Design review of the part built by this model. Coordinates are the model's own, in mm. A direction names the side the tool comes from. Coordinates: 2 decimals unless noted, no trailing zeros. Loops run counter-clockwise (first coordinate to the right, second up) from the corner with the lowest first, then second, coordinate; pieces in that order, holes last. Notation, with made-up numbers: (64.25, -2) - (109.25, -2) arc R28 cw to (109.25, 31) - close; hole circle Ø3 at (81, 63.25). An arc over 180 degrees is marked (long way). Use one line per item in the form item = value. Start each with the question number.
(1) Clearance check with flat-ended pins moving along their axes: pin 1 Ø1.3 at (x, y) = (-11.93, 18.67) entering from -Z; pin 2 Ø0.6 at (x, z) = (4.5, 1) entering from -Y; pin 3 Ø2 at (x, y) = (7.5, -21) entering from -Z. State where each tip first meets the part, or that it passes through.
(2) Add section D-D (y = -56.75). State the section outline as (x, z) points.
(3) Add section B-B (z = 0.55). Count the separate pieces of the cut face and the enclosed holes in it, plus the area to 3 significant figures.
(4) Tool access review of faces 5 (the face through (8.1, -19.5, 1.5)), 6 (the face through (-8.41, -5.83, 1.01)), 7 (the face through (-15.75, -11, 1)): name each direction out of +Z, -Z, +X, -X, +Y, -Y from which nothing blocks a thin tool from reaching the whole face with its end or side.
(5) Add section A-A (y = 10.65). State the section outline as (x, z) points, plus the area to 3 significant figures.
(6) The part is to be moulded in two halves that separate along Y. For faces 1 (the face through (10.655, -49.735, 1.493)), 2 (the face through (15.75, -10, 1)), 3 (the face through (-7, 11.5, 1)), 4 (the face through (0.22, 19.25, 0.99)), say which applies: pulls with the +Y half, pulls with the -Y half, needs draft (parallel to the pull), parting line crosses it, or undercut.
(7) For L1, parallel to X at y = 10.5, z = 1.8; L2, parallel to X at y = -40.5, z = 0.5; L3, parallel to Y at x = -3.5, z = 1.3, list the stretches that pass through material, from the lowest coordinate up.
Autodesk Inventor part; units mm, degrees
ref_plane "YZ Plane" through (0, 0, 0) normal (1, 0, 0) x (0, 1, 0)
ref_plane "XZ Plane" through (0, 0, 0) normal (0, 1, 0) x (-1, 0, 0)
ref_plane "XY Plane" through (0, 0, 0) normal (0, 0, 1) x (1, 0, 0)
sketch "スケッチ1" plane through (0, 0, 0) normal (0, 0, 1) x (1, 0, 0)
  circle A0 centre (-10.8253, -50.5) radius 0.7835
  circle A1 centre (0, -56.75) radius 0.7835
  circle A2 centre (10.8253, -50.5) radius 0.7835
  circle A3 centre (11.9284, 18.6695) radius 0.7835
  circle A4 centre (0, 16.025) radius 0.7835
  circle A5 centre (-11.9284, 18.6695) radius 0.7835
  line L0 (-9.85, -18.05) -> (-9.85, -7.35)
  arc A6 (-6.8, 12.8) -> (-9.85, 9.75) centre (-6.8, 9.75) ccw
  line L1 (-6.8, 12.8) -> (6.8, 12.8)
  arc A7 (9.85, 9.75) -> (6.8, 12.8) centre (6.8, 9.75) ccw
  line L2 (9.85, 9.75) -> (9.85, 8.57)
  arc A8 (4.8, -23.1) -> (9.85, -18.05) centre (4.8, -18.05) ccw
  line L3 (4.8, -23.1) -> (-4.8, -23.1)
  arc A9 (-9.85, -18.05) -> (-4.8, -23.1) centre (-4.8, -18.05) ccw
  circle A10 centre (0, -44.25) radius 4
  arc A11 (-15.75, 24.8351) -> (15.75, 24.8351) centre (0, 44.25) ccw
  line L4 (-15.75, -44.25) -> (-15.75, 24.8351)
  arc A12 (-15.75, -44.25) -> (15.75, -44.25) centre (0, -44.25) ccw
  line L5 (15.75, 24.8351) -> (15.75, -44.25)
  line L6 (-9.85, 8.57) -> (9.85, 8.57)
  line L7 (9.85, 8.57) -> (9.85, -7.35)
  line L8 (9.85, -7.35) -> (-9.85, -7.35)
  line L9 (-9.85, -7.35) -> (-9.85, 8.57)
  line L10 (9.85, 8.57) -> (9.85, -7.35)
  line L11 (-9.85, 8.57) -> (-9.85, 9.75)
  line L12 (-9.85, -7.35) -> (-9.85, 8.57)
  line L13 (9.85, -7.35) -> (9.85, -18.05)
  point P0 (0, 0)
  point P1 (0, 0)
  dimension "d3" = 4.23
  dimension "d4" = 15.75
extrude "押し出し2" add sketch "スケッチ1" along normal blind 2 contours L0 L8 L13 A8 L3 A9 | L11 A6 L1 A7 L2 L6 | A11 L5 A12 L4
sketch "スケッチ2" plane through (0, 0, 2) normal (0, 0, 1) x (1, 0, 0)
  line L0 (9.85, -7.35) -> (-9.85, -7.35)
  line L1 (15.75, 24.8351) -> (15.75, -44.25)
  line L2 (-15.75, -44.25) -> (-15.75, 24.8351)
  line L3 (0, 18.6695) -> (0, -60)
  point P0 (0, 0)
  point P1 (0, 0)
  point P2 (-7.7, 10.65)
  point P3 (-7.2, -20.45)
  point P4 (7.2, -20.45)
  point P5 (7.7, 10.65)
  point P6 (0, -14.25)
  dimension "d10" = 31.1
  dimension "d11" = 31.1
  dimension "d12" = 15.4
  dimension "d13" = 14.4
  dimension "d14" = 15.4
  dimension "d15" = 31.5
  dimension "d16" = 14.4
  dimension "d26" = 6.9
  dimension "d27" = 6.2
  dimension "d28" = 6.2
hole "Hole2" at (7.7, 10.65, 2) at (7.2, -20.45, 2) at (-7.2, -20.45, 2) at (-7.7, 10.65, 2) at (0, -14.25, 2) direction (0, 0, -1) diameter 2.2 depth 8 tip angle 118
sketch "スケッチ4" plane through (0, 0, 2) normal (0, 0, 1) x (1, 0, 0)
  point P0 (0, 0)
  point P1 (0, -14.25)
hole "Hole3" at (0, -14.25, 2) direction (0, 0, -1) diameter 9 depth 8 tip angle 118
fillet "フィレット3" radius 1.05 2 edges at (-9.85, 8.57, 1) (9.85, 8.57, 1)
fillet "フィレット4" radius 5.05 2 edges at (-9.85, -7.35, 1) (9.85, -7.35, 1)
sketch "スケッチ6" plane through (0, 0, 0) normal (0, 0, -1) x (-1, 0, 0)
  circle A0 centre (-10.8253, -50.5) radius 0.7835
  circle A1 centre (0, -56.75) radius 0.7835
  circle A2 centre (10.8253, -50.5) radius 0.7835
  circle A3 centre (0, -44.25) radius 10.5
  circle A4 centre (0, -44.25) radius 14.5
  point P0 (0, 0)
  dimension "d50" = 21
  dimension "d51" = 29
extrude "押し出し4" cut sketch "スケッチ6" against normal blind 1
fillet "フィレット5" radius 0.5 2 edges at (-15.75, 24.8351, 1) (15.75, 24.8351, 1)
sketch "スケッチ8" plane through (0, 0, 0) normal (0, 0, -1) x (-1, 0, 0)
  circle A0 centre (-7.2, -20.45) radius 1.1
  circle A1 centre (7.2, -20.45) radius 1.1
  point P0 (0, 0)
hole "Hole5" at (7.2, -20.45, 0) at (-7.2, -20.45, 0) direction (0, 0, 1) diameter 4.2 depth 1.5
sketch "スケッチ9" plane through (0, -44.25, 0) normal (0, 0, -1) x (-1, 0, 0)
  circle A0 centre (0, 0) radius 4
  circle A1 centre (0, 0) radius 3
  point P0 (0, 44.25)
  dimension "d69" = 6
extrude "押し出し6" add sketch "スケッチ9" against normal blind 2
properties part number "JointC2cover_2nd"
Computed values:
q1.pin_1 = through
q1.pin_2 = -59.43
q1.pin_3 = 1.5
q2.outline = (-9.58, 0) - (-7.35, 0) - (-7.35, 1) - (-0.78, 1) - (-0.78, 2) - (-9.58, 2) - close; (0.78, 1) - (7.35, 1) - (7.35, 0) - (9.58, 0) - (9.58, 2) - (0.78, 2) - close
q3.separate_pieces = 2
q3.enclosed_holes = 11
q3.area = 1,700 mm^2
q4.face_5 = -Z
q4.face_6 = +Z, -Z
q4.face_7 = +Z, -Z, -X, +Y, -Y
q5.outline = (-15.75, 0) - (-8.8, 0) - (-8.8, 2) - (-15.75, 2) - close; (-6.6, 0) - (6.6, 0) - (6.6, 2) - (-6.6, 2) - close; (8.8, 0) - (15.75, 0) - (15.75, 2) - (8.8, 2) - close
q5.area = 54.2 mm^2
q6.face_1 = undercut
q6.face_2 = needs draft
q6.face_3 = undercut
q6.face_4 = pulls with the +Y half
q7.L1 = -15.75 to -8.79, -6.61 to 6.61, 8.79 to 15.75
q7.L2 = -15.75 to -14.01, -9.81 to 9.81, 14.01 to 15.75
q7.L3 = -59.61 to -17.08, -11.42 to -7.35, 8.57 to 19.5
